For this review, take the finished solid that the model builds, in its own axes (mm). A direction names the side the tool comes from. Give positions to 0.01 mm unless a question says otherwise; leave off trailing zeros. Order: outer loops, then holes, each group sorted by start corner. A loop starts at its lowest first (then second) coordinate and runs counter-clockwise, first axis right, second up. Notation, with made-up numbers: (36.5, 20) - (75.5, 20) arc R10 ccw to (75.5, 36) - close; hole circle Ø1 at (44, -1.75). An arc over 180 degrees is marked (long way). Answer as a JSON object with one key per item and string values. Group by question number.
from build123d import *
from OCP.BRepFilletAPI import BRepFilletAPI_MakeChamfer

# Parameters (mm, degrees)
SKETCH2_W           = 192
SKETCH2_H           = 25
BOSS_EXTRUDE1_DEPTH = 8
SKETCH3_R           = 2.65
SKETCH3_R_2         = 2.25
CUT_EXTRUDE1_DEPTH  = 98.140362363
SKETCH5_W           = 16
SKETCH5_H           = 25.5
SKETCH5_R           = 2.65
BOSS_EXTRUDE2_DEPTH = 8
FILLET1_R           = 5
FILLET2_R           = 2
CHAMFER1_SIZE       = 1
CHAMFER1_SIZE2      = 1.732050808
CHAMFER2_SIZE       = 1
CHAMFER2_SIZE2      = 0.577350269


with BuildPart() as part:
    # Sketch2 → Boss-Extrude1 (new body)
    with BuildSketch(Plane.XY):
        Rectangle(SKETCH2_W, SKETCH2_H)
    extrude(amount=BOSS_EXTRUDE1_DEPTH)

    # Sketch3 → Cut-Extrude1 (cut, through all)
    with BuildSketch(Plane.XY.offset(8)):
        with Locations((-84, 0)):
            Circle(SKETCH3_R)
        with Locations((36.5, 0)):
            Circle(SKETCH3_R)
        with Locations((76.75, -3.5)):
            Circle(SKETCH3_R_2)
        with Locations((86.75, -3.5)):
            Circle(SKETCH3_R_2)
        with Locations((81.75, 4.5)):
            Circle(SKETCH3_R_2)
    extrude(amount=-CUT_EXTRUDE1_DEPTH, mode=Mode.SUBTRACT)

    # Sketch5 → Boss-Extrude2 (add)
    # profile 1 of 2: a face of its own
    with BuildSketch(Plane.XY.offset(8)):
        with Locations((-53.75, -25.25)):
            Rectangle(SKETCH5_W, SKETCH5_H)
        with Locations((-53.75, -30)):
            Circle(SKETCH5_R, mode=Mode.SUBTRACT)
    # profile 2 of 2: a face of its own
    with BuildSketch(Plane.XY.offset(8)):
        with Locations((6.25, -25.25)):
            Rectangle(SKETCH5_W, SKETCH5_H)
        with Locations(Location((6.25, -30, 0), (0, 0, 180))):
            Circle(SKETCH5_R, mode=Mode.SUBTRACT)
    extrude(amount=-BOSS_EXTRUDE2_DEPTH)

    # Fillet1
    fillet1_edges = [part.edges().sort_by_distance(p)[0] for p in [
        (-61.75, -38, 4),
        (-61.75, -12.5, 4),
        (-45.75, -12.5, 4),
        (-45.75, -38, 4),
        (14.25, -12.5, 4),
        (14.25, -38, 4),
        (-1.75, -38, 4),
        (-1.75, -12.5, 4),
        (96, -12.5, 4),
        (-96, -12.5, 4),
        (-96, 12.5, 4),
        (96, 12.5, 4),
    ]]
    fillet(fillet1_edges, radius=FILLET1_R)

    # Fillet2
    fillet2_edges = [part.edges().sort_by_distance(p)[0] for p in [
        (15.714466094, -13.964466094, 8),
        (-3.214466094, -13.964466094, 8),
        (-63.214466094, -13.964466094, 8),
        (-44.285533906, -13.964466094, 8),
        (14.25, -25.25, 8),
        (55.125, -12.5, 8),
        (6.25, -38, 8),
        (96, 0, 8),
        (0, 12.5, 8),
        (-96, 0, 8),
        (-78.875, -12.5, 8),
        (-61.75, -25.25, 8),
        (-53.75, -38, 8),
        (-45.75, -25.25, 8),
        (-23.75, -12.5, 8),
        (-1.75, -25.25, 8),
        (94.535533906, 11.035533906, 8),
        (94.535533906, -11.035533906, 8),
        (-94.535533906, 11.035533906, 8),
        (-94.535533906, -11.035533906, 8),
        (-47.214466094, -36.535533906, 8),
        (-60.285533906, -36.535533906, 8),
        (-0.285533906, -36.535533906, 8),
        (12.785533906, -36.535533906, 8),
    ]]
    fillet(fillet2_edges, radius=FILLET2_R)

    # Chamfer1
    chamfer1_edges = [part.edges().sort_by_distance(p)[0] for p in [
        (15.714466094, -13.964466094, 0),
        (-3.214466094, -13.964466094, 0),
        (-63.214466094, -13.964466094, 0),
        (-44.285533906, -13.964466094, 0),
        (14.25, -25.25, 0),
        (55.125, -12.5, 0),
        (6.25, -38, 0),
        (96, 0, 0),
        (-1.75, -25.25, 0),
        (-23.75, -12.5, 0),
        (-45.75, -25.25, 0),
        (-53.75, -38, 0),
        (-61.75, -25.25, 0),
        (-78.875, -12.5, 0),
        (-96, 0, 0),
        (0, 12.5, 0),
        (94.535533906, 11.035533906, 0),
        (94.535533906, -11.035533906, 0),
        (-94.535533906, 11.035533906, 0),
        (-94.535533906, -11.035533906, 0),
        (-47.214466094, -36.535533906, 0),
        (-60.285533906, -36.535533906, 0),
        (-0.285533906, -36.535533906, 0),
        (12.785533906, -36.535533906, 0),
    ]]
    chamfer1_side = [part.faces().sort_by_distance(p)[0] for p in [
        (-3.880983741, -3.433352853, 0),
    ]]
    chamfer(chamfer1_edges, length=CHAMFER1_SIZE, length2=CHAMFER1_SIZE2, reference=chamfer1_side[0])

    # Chamfer2: one chamfer whose edges measure the first distance from different faces: ONE call of the kernel's chamfer builder (chamfer() names one face for all edges)
    chamfer2_edges_1 = [part.edges().sort_by_distance(p)[0] for p in [
        (-86.65, 0, 0),
    ]]
    chamfer2_side_1 = [part.faces().sort_by_distance(p)[0] for p in [
        (-86.65, 0, 4),
    ]]
    chamfer2_edges_2 = [part.edges().sort_by_distance(p)[0] for p in [
        (33.85, 0, 0),
    ]]
    chamfer2_side_2 = [part.faces().sort_by_distance(p)[0] for p in [
        (33.85, 0, 4),
    ]]
    chamfer2_edges_3 = [part.edges().sort_by_distance(p)[0] for p in [
        (74.5, -3.5, 0),
    ]]
    chamfer2_side_3 = [part.faces().sort_by_distance(p)[0] for p in [
        (74.5, -3.5, 4),
    ]]
    chamfer2_edges_4 = [part.edges().sort_by_distance(p)[0] for p in [
        (84.5, -3.5, 0),
    ]]
    chamfer2_side_4 = [part.faces().sort_by_distance(p)[0] for p in [
        (84.5, -3.5, 4),
    ]]
    chamfer2_edges_5 = [part.edges().sort_by_distance(p)[0] for p in [
        (79.5, 4.5, 0),
    ]]
    chamfer2_side_5 = [part.faces().sort_by_distance(p)[0] for p in [
        (79.5, 4.5, 4),
    ]]
    chamfer2_edges_6 = [part.edges().sort_by_distance(p)[0] for p in [
        (-56.4, -30, 0),
    ]]
    chamfer2_side_6 = [part.faces().sort_by_distance(p)[0] for p in [
        (-56.4, -30, 4),
    ]]
    chamfer2_edges_7 = [part.edges().sort_by_distance(p)[0] for p in [
        (8.9, -30, 0),
    ]]
    chamfer2_side_7 = [part.faces().sort_by_distance(p)[0] for p in [
        (8.9, -30, 4),
    ]]
    chamfer2 = BRepFilletAPI_MakeChamfer(part.part.solid().wrapped)
    for e in chamfer2_edges_1:
        chamfer2.Add(CHAMFER2_SIZE, CHAMFER2_SIZE2, e.wrapped, chamfer2_side_1[0].wrapped)  # the first distance lies on this face
    for e in chamfer2_edges_2:
        chamfer2.Add(CHAMFER2_SIZE, CHAMFER2_SIZE2, e.wrapped, chamfer2_side_2[0].wrapped)  # the first distance lies on this face
    for e in chamfer2_edges_3:
        chamfer2.Add(CHAMFER2_SIZE, CHAMFER2_SIZE2, e.wrapped, chamfer2_side_3[0].wrapped)  # the first distance lies on this face
    for e in chamfer2_edges_4:
        chamfer2.Add(CHAMFER2_SIZE, CHAMFER2_SIZE2, e.wrapped, chamfer2_side_4[0].wrapped)  # the first distance lies on this face
    for e in chamfer2_edges_5:
        chamfer2.Add(CHAMFER2_SIZE, CHAMFER2_SIZE2, e.wrapped, chamfer2_side_5[0].wrapped)  # the first distance lies on this face
    for e in chamfer2_edges_6:
        chamfer2.Add(CHAMFER2_SIZE, CHAMFER2_SIZE2, e.wrapped, chamfer2_side_6[0].wrapped)  # the first distance lies on this face
    for e in chamfer2_edges_7:
        chamfer2.Add(CHAMFER2_SIZE, CHAMFER2_SIZE2, e.wrapped, chamfer2_side_7[0].wrapped)  # the first distance lies on this face
    add(Compound.cast(chamfer2.Shape()), mode=Mode.REPLACE)


solid = part.part
1) For line 1 (X direction, y = -33.5, z = 3.75); line 2 (Y direction, x = -84, z = 4.25); line 3 (Y direction, x = 86.5, z = 1.75), list the stretches that pass through material, from the lowest coordinate up.
2) For pin 1 (4.5 mm diameter, centred on x = -76, z = 4, fed in from -Y); pin 2 (3.5 mm diameter, centred on y = -24, z = 3.5, fed in from +X); pin 3 (3 mm diameter, centred on y = -27.5, z = 4.5, fed in from -X); pin 4 (3 mm diameter, centred on x = 6.25, y = -30, fed in from +Z), all flat-tipped, find the tip position at first contact; note any pin that passes through.
3) Consider section A-A (x = 86.75). Give the boundary of the cut face in (y, z), plus the area to 3 significant figures.
4) Consider section D-D (x = 29). Give the boundary of the cut face in (y, z).
5) Mouldability with a two-part tool opening along Y and no side actions: class faces 6 (the face through (-1.75, -25, 4)), 7 (the face through (-59.824, -36.142, 0.686)), 8 (the face through (-81.472, 0.796, 4.549)) as released by +Y, released by -Y, zero draft, split by the parting line, or undercut.
6) For faces 1 (the face through (-2.9, -13.74, 1.07)), 2 (the face through (-24, -12.5, 4)), 3 (the face through (15.49, -13.65, 1.07)), 4 (the face through (14.25, -25, 4)), 5 (the face through (78.83, -4.36, 4.55)), list the 3-axis set-ups (+Z, -Z, +X, -X, +Y, -Y) from which the entire face can be reached by the end or side of a thin tool; tool diameter is ignored.
7) Consider section C-C (z = 3.25). Give the number of separate pieces and of enclosed holes in the cut face, plus the area to 3 significant figures.
8) Consider section B-B (y = -30). Give the boundary of the cut face in (x, z).
Result set:
{
 "1": {"line 1": "x = -61.72 to -45.78, -1.72 to 14.22", "line 2": "y = -12.5 to -2.65, 2.65 to 12.5", "line 3": "y = -12.5 to -5.74, -1.26 to 12.5"},
 "2": {"pin 1": "stops at y = -12.5", "pin 2": "stops at x = 14.25", "pin 3": "stops at x = -61.75", "pin 4": "passes through"},
 "3": {"outline": "(-12.5, 1.73) - (-11.5, 0) - (-6.33, 0) - (-5.75, 1) - (-5.75, 8) - (-10.5, 8) arc R2 ccw to (-12.5, 6) - close; (-1.25, 1) - (-0.67, 0) - (11.5, 0) - (12.5, 1.73) - (12.5, 6) arc R2 ccw to (10.5, 8) - (-1.25, 8) - close", "area": "160 mm2"},
 "4": {"outline": "(-12.5, 1.73) - (-11.5, 0) - (11.5, 0) - (12.5, 1.73) - (12.5, 6) arc R2 ccw to (10.5, 8) - (-10.5, 8) arc R2 ccw to (-12.5, 6) - close"},
 "5": {"face 6": "zero draft", "face 7": "released by -Y", "face 8": "undercut"},
 "6": {"face 1": "-Z, -Y", "face 2": "+Z, -Z, -Y", "face 3": "-Z, +X, -Y", "face 4": "+Z, -Z, +X, -Y", "face 5": "+Z, -Z"},
 "7": {"separate pieces": "1", "enclosed holes": "7", "area": "5,460 mm2"},
 "8": {"outline": "(-61.75, 1.73) - (-60.75, 0) - (-56.98, 0) - (-56.4, 1) - (-56.4, 8) - (-59.75, 8) arc R2 ccw to (-61.75, 6) - close; (-51.1, 1) - (-50.52, 0) - (-46.75, 0) - (-45.75, 1.73) - (-45.75, 6) arc R2 ccw to (-47.75, 8) - (-51.1, 8) - close; (-1.75, 1.73) - (-0.75, 0) - (3.02, 0) - (3.6, 1) - (3.6, 8) - (0.25, 8) arc R2 ccw to (-1.75, 6) - close; (8.9, 1) - (9.48, 0) - (13.25, 0) - (14.25, 1.73) - (14.25, 6) arc R2 ccw to (12.25, 8) - (8.9, 8) - close"}
}
